Input: part model. Units: mm. Frame: model coordinates. Face numbers are marked on the shaded views. A direction names the side the tool comes from. Give positions to 0.01 mm unless a question says otherwise; leave off trailing zeros. Write each loop counter-clockwise with the first axis right and the second up, starting at its lowest first coordinate (ties: lowest second). Pieces come first, ordered by that corner, then holes.
```python
from build123d import *

# Parameters (mm, degrees)
SKETCH2_R           = 2.3
SKETCH2_R_2         = 0.6
BOSS_EXTRUDE1_DEPTH = 3


with BuildPart() as part:
    # Sketch2 → Boss-Extrude1 (new body)
    with BuildSketch(Plane.XY):
        with BuildLine():
            Line((16.770369268, 4.5), (46.770369268, 4.5))
            ThreePointArc((46.770369268, 4.5), (51.270370099, 0), (46.770369268, -4.5))
            Line((46.770369268, -4.5), (24.560820229, -4.5))
            ThreePointArc((24.560820229, -4.5), (24.371598614, -4.635229787), (24.438260986, -4.858048195))
            Line((24.438260986, -4.858048195), (27.065199516, -6.895120487))
            ThreePointArc((27.065199516, -6.895120487), (27.209672091, -6.973054037), (27.371597624, -7))
            Line((27.371597624, -7), (46.770368806, -7))
            ThreePointArc((46.770368806, -7), (53.770370099, -2.31e-07), (46.770369268, 7))
            Line((46.770369268, 7), (1.770370099, 7))
            ThreePointArc((1.770370099, 7), (-5.229629901, 0), (1.770370099, -7))
            Line((1.770370099, -7), (17.871597624, -7))
            ThreePointArc((17.871597624, -7), (18.057004855, -6.874994391), (18.010642647, -6.656241586))
            Line((18.010642647, -6.656241586), (14.012786293, -3.556084383))
            ThreePointArc((14.012786293, -3.556084383), (12.512882937, 1.457329797), (16.770369268, 4.5))
        make_face()
        with Locations((3.520369683, 0)):
            Circle(SKETCH2_R, mode=Mode.SUBTRACT)
        with Locations((8.370369683, 0)):
            Circle(SKETCH2_R_2, mode=Mode.SUBTRACT)
        with Locations((10.370369683, 0)):
            Circle(SKETCH2_R_2, mode=Mode.SUBTRACT)
        with Locations((-0.929630317, 0)):
            Circle(SKETCH2_R_2, mode=Mode.SUBTRACT)
        with Locations((-2.929630317, 0)):
            Circle(SKETCH2_R_2, mode=Mode.SUBTRACT)
    extrude(amount=BOSS_EXTRUDE1_DEPTH)


solid = part.part
```
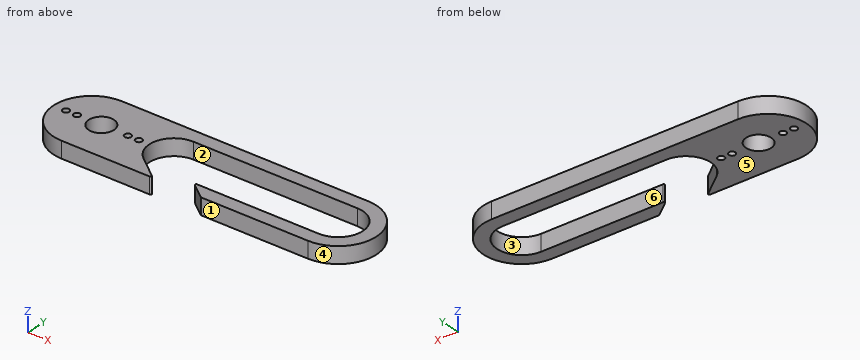
Item 1: Section B-B (z = 2.55). Return loops of the section in (x, y), and give its area (3 significant figures).
Item 2: Section D-D (x = 23.5). Return loops of the section in (y, z).
Item 3: Set-up query: the marked faces 1 and 2. Return all of +Z, -Z, +X, -X, +Y, -Y with unobstructed straight access to the full face (end or side cutting, diameter ignored); none if empty.
Item 4: Section A-A (x = 36). Return loops of the section in (y, z), and give its area (3 significant figures).
Item 5: Section C-C (y = 0). Return loops of the section in (x, z), and give its area (3 significant figures).
Item 6: Pin query (flat end, axial travel): pin 1 (1.4 mm diameter, centred on x = 10.37, y = 0, fed in from -Z); pin 2 (4 mm diameter, centred on x = 3.52, y = 0, fed in from -Z); pin 3 (1 mm diameter, centred on y = -4.5, z = 0.5, fed in from -X). Return the tip coordinate at first contact, or that it passes through.
Item 7: Ray query, line 1 (Y direction, x = 46.5, z = 1.15); line 2 (X direction, y = -1.25, z = 2.1); line 3 (Y direction, x = -0.5, z = 0.8). Return the intervals inside material, ascending.
Item 8: Mould query, pull axis Y, two halves, no side actions, for the marked faces 3, 4, 5 and 6. Classes: +Y half, -Y half, draft (parallel to the pull), parting line (faces both ways), or undercut.
Solved:
1. outline: (1.77, -7) - (17.87, -7) arc R0.2 ccw to (18.01, -6.66) - (14.01, -3.56) arc R4.5 cw to (16.77, 4.5) - (46.77, 4.5) arc R4.5 cw to (46.77, -4.5) - (24.56, -4.5) arc R0.2 ccw to (24.44, -4.86) - (27.07, -6.9) arc R0.5 ccw to (27.37, -7) - (46.77, -7) arc R7 ccw to (46.77, 7) - (1.77, 7) arc R7 ccw to start; hole circle Ø1.2 at (-2.93, 0); hole circle Ø1.2 at (-0.93, 0); hole circle Ø4.6 at (3.52, 0); hole circle Ø1.2 at (8.37, 0); hole circle Ø1.2 at (10.37, 0)
1. area: 407 mm2
2. outline: (4.5, 0) - (7, 0) - (7, 3) - (4.5, 3) - close
3. face 1: +Z, -Z, +X, -X, -Y
3. face 2: +Z, -Z
4. outline: (-7, 0) - (-4.5, 0) - (-4.5, 3) - (-7, 3) - close; (4.5, 0) - (7, 0) - (7, 3) - (4.5, 3) - close
4. area: 15.0 mm2
5. outline: (-5.23, 0) - (-3.53, 0) - (-3.53, 3) - (-5.23, 3) - close; (-2.33, 0) - (-1.53, 0) - (-1.53, 3) - (-2.33, 3) - close; (-0.33, 0) - (1.22, 0) - (1.22, 3) - (-0.33, 3) - close; (5.82, 0) - (7.77, 0) - (7.77, 3) - (5.82, 3) - close; (8.97, 0) - (9.77, 0) - (9.77, 3) - (8.97, 3) - close; (10.97, 0) - (12.27, 0) - (12.27, 3) - (10.97, 3) - close; (51.27, 0) - (53.77, 0) - (53.77, 3) - (51.27, 3) - close
5. area: 31.8 mm2
6. pin 1: stops at z = 0
6. pin 2: passes through
6. pin 3: stops at x = -3.97
7. line 1: y = -7 to -4.5, 4.5 to 7
7. line 2: x = -5.12 to 1.59, 5.45 to 12.45, 51.09 to 53.66
7. line 3: y = -6.62 to -0.42, 0.42 to 6.62
8. face 3: undercut
8. face 4: parting line
8. face 5: draft
8. face 6: undercut
